from build123d import *

# Parameters (mm, degrees)
SKETCH1_W           = 115
SKETCH1_H           = 70
BOSS_EXTRUDE1_DEPTH = 3
SKETCH2_W           = 109
SKETCH2_H           = 64
BOSS_EXTRUDE2_DEPTH = 3
FILLET1_R           = 2
SKETCH4_W           = 87.172440104
SKETCH4_H           = 51.155574538
CUT_EXTRUDE1_DEPTH  = 0.1


with BuildPart() as part:
    # Sketch1 → Boss-Extrude1 (new body)
    with BuildSketch(Plane(origin=(0, 0, 0), x_dir=(1, 0, 0), z_dir=(0, 1, 0))):
        Rectangle(SKETCH1_W, SKETCH1_H)
    extrude(amount=BOSS_EXTRUDE1_DEPTH)

    # Sketch2 → Boss-Extrude2 (add)
    with BuildSketch(Plane.XZ):
        Rectangle(SKETCH2_W, SKETCH2_H)
    extrude(amount=BOSS_EXTRUDE2_DEPTH)

    # Fillet1
    fillet1_edges = [part.edges().sort_by_distance(p)[0] for p in [
        (-57.5, 3, 0),
        (0, 3, 35),
        (57.5, 3, 0),
        (0, 3, -35),
        (57.5, 1.5, 35),
        (-57.5, 1.5, 35),
        (-57.5, 1.5, -35),
        (57.5, 1.5, -35),
    ]]
    fillet(fillet1_edges, radius=FILLET1_R)

    # Sketch4 → Cut-Extrude1 (cut)
    with BuildSketch(Plane(origin=(0, 3, 0), x_dir=(1, 0, 0), z_dir=(0, 1, 0))):
        Rectangle(SKETCH4_W, SKETCH4_H)
    extrude(amount=-CUT_EXTRUDE1_DEPTH, mode=Mode.SUBTRACT)


solid = part.part
Source: CAD feature listing. Evaluate the final solid. Frame: model axes, mm. A direction names the side the tool comes from. Coordinates: 2 decimals unless noted, no trailing zeros. Loops run counter-clockwise (first coordinate to the right, second up) from the corner with the lowest first, then second, coordinate; pieces in that order, holes last. Notation, with made-up numbers: (7.25, 70) - (35.25, 70) arc R31 cw to (35.25, 97) - close; hole circle Ø3 at (-29, -24). An arc over 180 degrees is marked (long way). Return JSON: item names as keys, results as strings.
Q1. Section C-C, the plane y = -1.5. Return loops of the section in (x, z), plus the area to 3 significant figures.
Results:
{"outline": "(-54.5, -32) - (54.5, -32) - (54.5, 32) - (-54.5, 32) - close", "area": "6,980 mm2"}
Q2. Section A-A, the plane x = -5.5. Return loops of the section in (y, z), plus the area to 3 significant figures.
Results:
{"outline": "(-3, -32) - (0, -32) - (0, -35) - (1, -35) arc R2 ccw to (3, -33) - (3, -25.58) - (2.9, -25.58) - (2.9, 25.58) - (3, 25.58) - (3, 33) arc R2 ccw to (1, 35) - (0, 35) - (0, 32) - (-3, 32) - close", "area": "395 mm2"}
Q3. Access query for faces 1 (the flat face through (-1, -1, -32)), 2 (the flat face through (-1, -1, 32)), 3 (the flat face through (-1, -3, 0)). Directions: +Z, -Z, +X, -X, +Y, -Y. A direction counts if a zero-diameter tool reaches every point of the face in a straight line with its end or side. Return the directions, or none.
Results:
{"face 1": "-Z, +X, -X, -Y", "face 2": "+Z, +X, -X, -Y", "face 3": "+Z, -Z, +X, -X, -Y"}
Q4. Mould query, pull axis X, two halves, no side actions, for faces 4 (the flat face through (-54.5, -1, 0)), 5 (the flat face through (-1, 3, 29)), 6 (the flat face through (-1, 2.9, 0)), 7 (the flat face through (54.5, -1, 0)). Classes: released by +X, released by -X, zero draft, split by the parting line, or undercut.
Results:
{"face 4": "released by -X", "face 5": "zero draft", "face 6": "undercut", "face 7": "released by +X"}
Q5. Section B-B, the plane z = -7. Return loops of the section in (x, y).
Results:
{"outline": "(-57.5, 0) - (-54.5, 0) - (-54.5, -3) - (54.5, -3) - (54.5, 0) - (57.5, 0) - (57.5, 1) arc R2 ccw to (55.5, 3) - (43.59, 3) - (43.59, 2.9) - (-43.59, 2.9) - (-43.59, 3) - (-55.5, 3) arc R2 ccw to (-57.5, 1) - close"}
Q6. Contact query for flat-ended pins moving along their axis: P1, Ø1.5, axis at x = -22, y = 2, coming from the -Z side; P2, Ø2.5, axis at y = -2, z = -10, coming from the +X side; P3, Ø1.5, axis at x = 18, y = -2, coming from the +Z side. Output: stop coordinate, or through.
Results:
{"P1": "z = -34.98", "P2": "x = 54.5", "P3": "z = 32"}
Q7. Material intervals for line 1 along Z through (x, y) = (34, -2.3); line 2 along Y through (x, z) = (14.5, -5); line 3 along X through (y, z) = (-2.7, -13), sorted ascending.
Results:
{"line 1": "-32 to 32", "line 2": "-3 to 2.9", "line 3": "-54.5 to 54.5"}
